```python
from build123d import *

# Parameters (mm, degrees)
F0_R     = 16.4973
F1_DEPTH = 3.9878
F2_R     = 0.7874
F3_R     = 1.5875
F4_DEPTH = 25.4


with BuildPart() as f1:
    # F0 (on Front) → F1 (new body)
    with BuildSketch(Plane.XZ):
        with Locations((-24.256999, 23.241002)):
            Circle(F0_R)
    extrude(amount=F1_DEPTH)

    # F2
    f2_edges = [f1.edges().sort_by_distance(p)[0] for p in [
        (-40.754299, 0, 23.241002),
        (-40.754299, -3.9878, 23.241002),
    ]]
    fillet(f2_edges, radius=F2_R)

    # F3 (on face) → F4 (cut)
    with BuildSketch(Plane.XZ.offset(3.9878)):
        with Locations((-24.257001, 35.179)):
            Circle(F3_R)
    extrude(amount=-F4_DEPTH, mode=Mode.SUBTRACT)


solid = f1.part
```
Verification items for the finished model (mm, model axes). Round coordinates to 2 decimals unless told otherwise and drop trailing zeros. Order: outer loops, then holes, each group sorted by start corner. A loop starts at its lowest first (then second) coordinate and runs counter-clockwise, first axis right, second up. Notation, with made-up numbers: (-13, 3.25) -> (19, 3.25) arc R11 cw to (19, 7.25) -> close; hole circle Ø4 at (82, 84). An arc over 180 degrees is marked (long way). Put each result on its own line as item: value. Start each with the question number.
(1) Material ranges on line 1 along Y through (x, z) = (-8.5, 24.5); line 2 along Z through (x, y) = (-22, -2.1); line 3 along Z through (x, y) = (-36.5, -1.15), recorded low to high.
(2) Depth check by flat-ended pin: pin 1 Ø3 at (x, z) = (-12, 10.5) entering from -Y; pin 2 Ø1 at (y, z) = (-3.5, 36) entering from +X; pin 3 Ø2 at (y, z) = (-1, 13) entering from -X. Enter the tip coordinate at first touch or a pass-through.
(3) Draft check along X on faces 1 (the face through (-24.6, -2.02, 33.63)), 2 (the face through (-15.388, -1.977, 37.152)), 3 (the face through (-24, -3.988, 23)). Enter one of: +X half, -X half, draft (parallel to the pull), parting line (faces both ways), or undercut.
(4) Section check A-A (y = -2.2). Enter the section's corners in (x, z) (1 decimal).
Completed:
1. line 1: y = -3.98 to -0.01
1. line 2: z = 6.9 to 39.58
1. line 3: z = 12.18 to 34.3
2. pin 1: stops at y = -3.83
2. pin 2: stops at x = -13.26
2. pin 3: stops at x = -37.92
3. face 1: undercut
3. face 2: parting line
3. face 3: draft
4. outline: circle Ø33 at (-24.3, 23.2); hole circle Ø3.2 at (-24.3, 35.2)
